```python
from build123d import *

# Parameters (mm, degrees)
BASE_FLANGE1_DEPTH = 0.2


# Sheet-metal steps are written as plain solids
with BuildPart() as part:
    # Sketch1 → Base-Flange1 (new body)
    with BuildSketch(Plane.XY):
        with BuildLine():
            Line((7.416198487, 3), (10.416198487, 3))
            Line((10.416198487, 3), (10.416198487, -3))
            Line((10.416198487, -3), (7.416198487, -3))
            ThreePointArc((7.416198487, -3), (0, -8), (-7.416198487, -3))
            Line((-7.416198487, -3), (-10.416198487, -3))
            Line((-10.416198487, -3), (-10.416198487, 3))
            Line((-10.416198487, 3), (-7.416198487, 3))
            ThreePointArc((-7.416198487, 3), (0, 8), (7.416198487, 3))
        make_face()
        with BuildLine():
            Line((-4.25, 3), (-4.25, -3))
            ThreePointArc((-4.25, -3), (0, -5), (4.25, -3))
            Line((4.25, -3), (4.25, 3))
            ThreePointArc((4.25, 3), (0, 5), (-4.25, 3))
        make_face(mode=Mode.SUBTRACT)
    extrude(amount=-BASE_FLANGE1_DEPTH)


solid = part.part
```
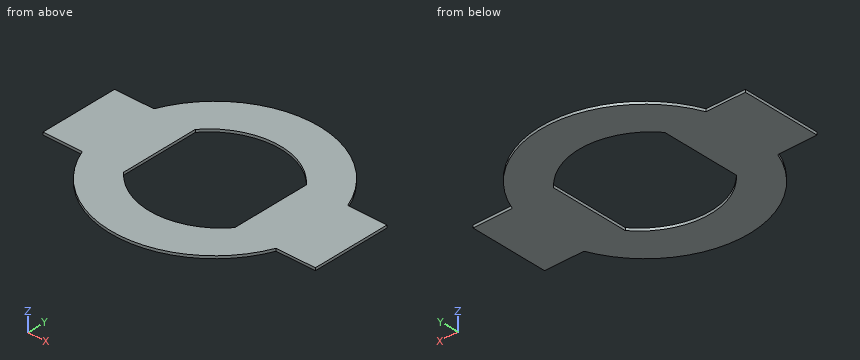
Can you work these out from the model? Positions are in its coordinate system, mm. Give positions to 0.01 mm unless a question says otherwise; leave off trailing zeros. Write each loop counter-clockwise with the first axis right and the second up, starting at its lowest first coordinate (ties: lowest second). Pieces come first, ordered by that corner, then holes. Notation, with made-up numbers: (68.25, 10.5) - (124.25, 10.5) arc R19 ccw to (124.25, 37.5) - close; hole circle Ø1 at (85, 2). An arc over 180 degrees is marked (long way). Write item = value, one per line. Start each with the question number.
1. Imagine slicing it at C-C (x = -2.25). Please give me the cut outline in (y, z), and give its area (3 significant figures).
2. Imagine slicing it at A-A (y = -2.25). Please give me the cut outline in (x, z), and give its area (3 significant figures).
3. Please list where these lines run through material, in increasing order: line 1 (X direction, y = -1, z = -0.05); line 2 (Y direction, x = 0.25, z = -0.1); line 3 (Y direction, x = -3.75, z = -0.15).
4. Imagine slicing it at D-D (x = 9.25). Please give me the cut outline in (y, z).
5. Imagine slicing it at B-B (z = -0.05). Please give me the cut outline in (x, y).
Worked answers:
q1.outline = (-7.68, -0.2) - (-4.52, -0.2) - (-4.52, 0) - (-7.68, 0) - close; (4.52, -0.2) - (7.68, -0.2) - (7.68, 0) - (4.52, 0) - close
q1.area = 1.26 mm2
q2.outline = (-10.42, -0.2) - (-4.25, -0.2) - (-4.25, 0) - (-10.42, 0) - close; (4.25, -0.2) - (10.42, -0.2) - (10.42, 0) - (4.25, 0) - close
q2.area = 2.47 mm2
q3.line_1 = -10.42 to -4.25, 4.25 to 10.42
q3.line_2 = -8 to -4.99, 4.99 to 8
q3.line_3 = -7.07 to -3.53, 3.53 to 7.07
q4.outline = (-3, -0.2) - (3, -0.2) - (3, 0) - (-3, 0) - close
q5.outline = (-10.42, -3) - (-7.42, -3) arc R8 ccw to (7.42, -3) - (10.42, -3) - (10.42, 3) - (7.42, 3) arc R8 ccw to (-7.42, 3) - (-10.42, 3) - close; hole (-4.25, -3) arc R5.52 ccw to (4.25, -3) - (4.25, 3) arc R5.52 ccw to (-4.25, 3) - close
